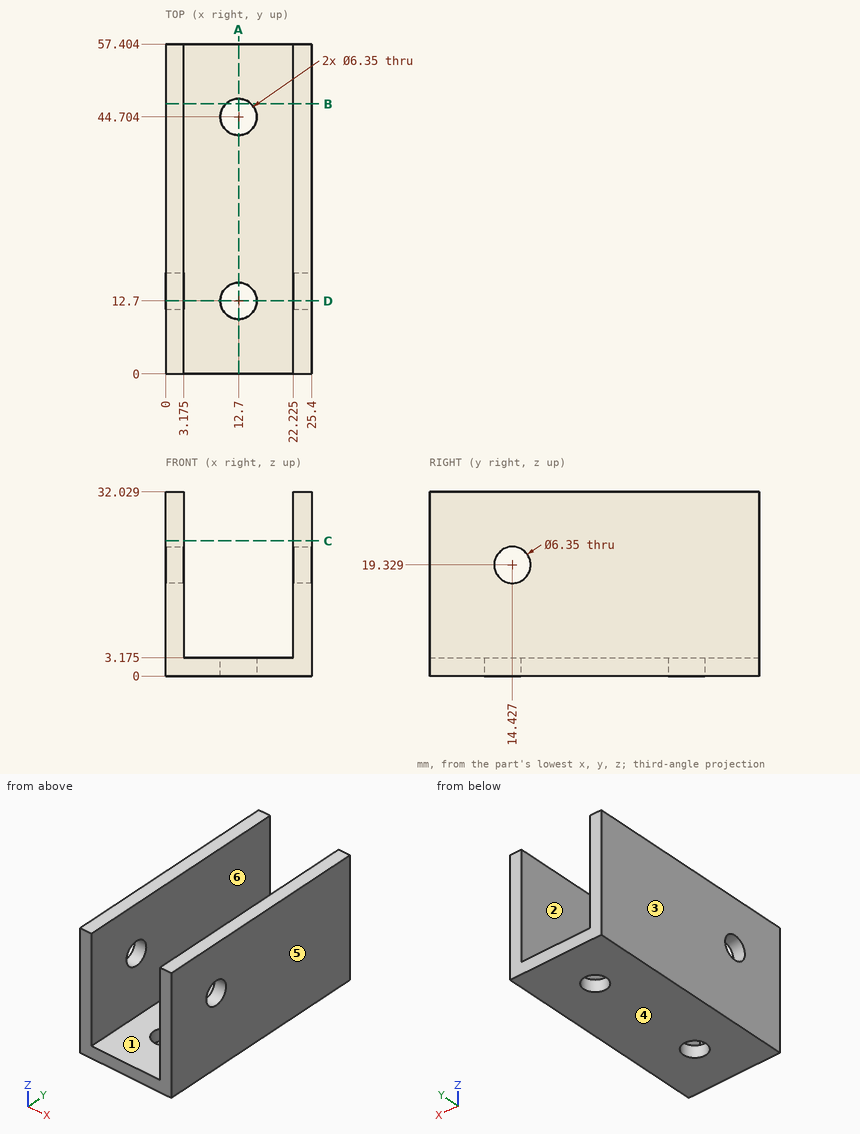
For this review, use the dimensioned drawing (mm, ordinates from the lowest corner) and the shaded views. A direction names the side the tool comes from. Give positions to 0.01 mm unless a question says otherwise; leave off trailing zeros. Write each loop counter-clockwise with the first axis right and the second up, starting at its lowest first coordinate (ties: lowest second). Pieces come first, ordered by that corner, then holes. Notation, with made-up numbers: M 53.25,2 L 75.25,2 A18 cw 75.25,34 Z; hole C 82.25,63 d9. An arc over 180 degrees is marked long. Answer as a JSON object with one key per item and string values. Group by question number.
Item 1: Consider section C-C on z = 23.5. Write out the cut boundary in (x, y) (1 decimal).
Item 2: Consider section A-A on x = 12.7. Write out the cut boundary in (y, z) (1 decimal).
Item 3: For probe 1 along Y at (x, z) = (12.7, 1.8) (1 decimal); probe 2 along X at (y, z) = (43, 10) (1 decimal); probe 3 along Z at (x, y) = (20.5, 28) (1 decimal), list the stretches that pass through material, from the lowest coordinate up. Write a range as [from, to].
Item 4: For pin 1 Ø7.5 at (y, z) = (14.43, 19.33) entering from +X; pin 2 Ø4 at (x, y) = (12.7, 12.7) entering from +Z; pin 3 Ø5.5 at (x, y) = (10, 18.5) entering from +Z (3 decimals), all flat-tipped, find the tip position at first contact; note any pin that passes through.
Item 5: Draft analysis for pull direction X (two halves, no side actions). For the marked faces 1, 2, 3 and 4, state which applies: +X half, -X half, draft (parallel to the pull), parting line (faces both ways), or undercut.
Item 6: Tool access review of the marked faces 5 and 6: name each direction out of +Z, -Z, +X, -X, +Y, -Y from which nothing blocks a thin tool from reaching the whole face with its end or side.
Item 7: Consider section D-D on y = 12.7. Write out the cut boundary in (x, z) (1 decimal), plus the area to 3 significant figures.
Item 8: Consider section B-B on y = 47. Write out the cut boundary in (x, z) (1 decimal).
Check result:
{
 "1": {"outline": "M 0,0 L 3.2,0 L 3.2,57.4 L 0,57.4 Z; M 22.2,0 L 25.4,0 L 25.4,57.4 L 22.2,57.4 Z"},
 "2": {"outline": "M 0,0 L 9.5,0 L 9.5,3.2 L 0,3.2 Z; M 15.9,0 L 41.5,0 L 41.5,3.2 L 15.9,3.2 Z; M 47.9,0 L 57.4,0 L 57.4,3.2 L 47.9,3.2 Z"},
 "3": {"probe 1": "y = [0, 9.5], [15.9, 41.5], [47.9, 57.4]", "probe 2": "x = [0, 3.2], [22.2, 25.4]", "probe 3": "z = [0, 3.2]"},
 "4": {"pin 1": "stops at x = 25.4", "pin 2": "passes through", "pin 3": "stops at z = 3.175"},
 "5": {"face 1": "undercut", "face 2": "undercut", "face 3": "-X half", "face 4": "draft"},
 "6": {"face 5": "+Z, -Z, +X, +Y, -Y", "face 6": "+Z, +Y, -Y"},
 "7": {"outline": "M 0,0 L 9.5,0 L 9.5,3.2 L 3.2,3.2 L 3.2,16.7 L 0,16.7 Z; M 0,22 L 3.2,22 L 3.2,32 L 0,32 Z; M 15.9,0 L 25.4,0 L 25.4,16.7 L 22.2,16.7 L 22.2,3.2 L 15.9,3.2 Z; M 22.2,22 L 25.4,22 L 25.4,32 L 22.2,32 Z", "area": "210 mm^2"},
 "8": {"outline": "M 0,0 L 10.5,0 L 10.5,3.2 L 3.2,3.2 L 3.2,32 L 0,32 Z; M 14.9,0 L 25.4,0 L 25.4,32 L 22.2,32 L 22.2,3.2 L 14.9,3.2 Z"}
}
